```python
from build123d import *

# Parameters (mm, degrees)
SKETCH2_R           = 39.5
BOSS_EXTRUDE1_DEPTH = 1
SKETCH4_R           = 41.25
BOSS_EXTRUDE2_DEPTH = 1
SKETCH5_R           = 42
BOSS_EXTRUDE3_DEPTH = 7
SKETCH6_R           = 35
BOSS_EXTRUDE4_DEPTH = 7
BOSS_EXTRUDE5_DEPTH = 3
CIRPATTERN1_COUNT   = 12
SKETCH8_R           = 15
BOSS_EXTRUDE6_DEPTH = 10
SKETCH9_W           = 35
SKETCH9_H           = 40
BOSS_EXTRUDE7_DEPTH = 42
BOSS_EXTRUDE8_DEPTH = 35
SKETCH11_R          = 15
BOSS_EXTRUDE9_DEPTH = 10


with BuildPart() as part:
    # Sketch1 → Revolve1 (revolve)
    with BuildSketch(Plane.XY):
        with BuildLine():
            Line((-35, 0), (0, 0))
            Line((0, 0), (0, -20))
            Line((0, -20), (-40, -20))
            ThreePointArc((-40, -20), (-39.657515479, -9.46062113), (-35, 0))
        make_face()
    revolve(axis=Axis((0, 0, 0), (0, -1, 0)))

    # Sketch2 → Boss-Extrude1 (add)
    with BuildSketch(Plane.XZ.offset(20)):
        Circle(SKETCH2_R)
    extrude(amount=BOSS_EXTRUDE1_DEPTH)

    # Sketch3 → Revolve2 (revolve)
    with BuildSketch(Plane(origin=(0, 0, 0), x_dir=(0, 0, -1), z_dir=(1, 0, 0))):
        with BuildLine():
            Line((0, -21), (-40, -21))
            ThreePointArc((-40, -21), (-42.384109041, -30.861589096), (-42, -41))
            Line((-42, -41), (0, -41))
            Line((0, -41), (0, -21))
        make_face()
    revolve(axis=Axis((0, -21, 0), (0, -1, 0)))

    # Sketch4 → Boss-Extrude2 (add)
    with BuildSketch(Plane.XZ.offset(41)):
        Circle(SKETCH4_R)
    extrude(amount=BOSS_EXTRUDE2_DEPTH)

    # Sketch5 → Boss-Extrude3 (add)
    with BuildSketch(Plane.XZ.offset(42)):
        Circle(SKETCH5_R)
    extrude(amount=BOSS_EXTRUDE3_DEPTH)

    # Sketch6 → Boss-Extrude4 (add)
    with BuildSketch(Plane.XZ.offset(49)):
        Circle(SKETCH6_R)
    extrude(amount=BOSS_EXTRUDE4_DEPTH)

    # Sketch7 → Boss-Extrude5 (add)
    with BuildSketch(Plane.XZ.offset(49)):
        Polygon((40.75, 0), (39.625, 1.948557159), (37.375, 1.948557159), (36.25, 0), (37.375, -1.948557159), (39.625, -1.948557159), align=None)
        Polygon((39.047649731, 0.948557159), (37.952350269, 0.948557159), (37.404700538, 0), (37.952350269, -0.948557159), (39.047649731, -0.948557159), (39.595299462, 0), align=None, mode=Mode.SUBTRACT)
    boss_extrude5 = extrude(amount=BOSS_EXTRUDE5_DEPTH)

    # CirPattern1: Boss-Extrude5 ×12 about axis
    cirpattern1_axis = Axis((0, 0, 0), (0, 1, 0))
    for i in range(1, CIRPATTERN1_COUNT):
        add(boss_extrude5.rotate(cirpattern1_axis, i * 360 / CIRPATTERN1_COUNT))

    # Sketch8 → Boss-Extrude6 (add)
    with BuildSketch(Plane.XZ.offset(56)):
        Circle(SKETCH8_R)
    extrude(amount=BOSS_EXTRUDE6_DEPTH)

    # Sketch9 → Boss-Extrude7 (add)
    with BuildSketch(Plane(origin=(0, 0, 0), x_dir=(1, 0, 0), z_dir=(0, 1, 0))):
        Rectangle(SKETCH9_W, SKETCH9_H)
    extrude(amount=BOSS_EXTRUDE7_DEPTH)

    # Sketch10 → Boss-Extrude8 (add)
    with BuildSketch(Plane.ZY.offset(17.5)):
        with BuildLine():
            Line((-20, 42), (20, 42))
            ThreePointArc((20, 42), (0, 62), (-20, 42))
        make_face()
    extrude(amount=-BOSS_EXTRUDE8_DEPTH)

    # Sketch11 → Boss-Extrude9 (add)
    with BuildSketch(Plane.ZY.offset(17.5)):
        with Locations((0, 42)):
            Circle(SKETCH11_R)
    boss_extrude9 = extrude(amount=BOSS_EXTRUDE9_DEPTH)

    # Mirror1: Boss-Extrude9 across plane
    add(boss_extrude9.mirror(Plane(origin=(0, 0, 0), x_dir=(0, 0, 1), z_dir=(1, 0, 0))))


solid = part.part
```
Check sheet for the modelled part. Datum: model origin and axes. Units: mm. A direction names the side the tool comes from. Give positions to 0.01 mm unless a question says otherwise; leave off trailing zeros. Loops run counter-clockwise (first coordinate to the right, second up) from the corner with the lowest first, then second, coordinate; pieces in that order, holes last. Notation, with made-up numbers: M 18.5,84.5 L 39.5,84.5 A23 ccw 39.5,99.5 Z; hole C 65.25,56 d6. An arc over 180 degrees is marked long. Answer as CSV lines item,"result".
Item 1: Depth check by flat-ended pin: pin 1 Ø10 at (x, z) = (13, -17.5) entering from +Y; pin 2 Ø1.2 at (x, z) = (-32.5, 19.5) entering from -Y; pin 3 Ø3 at (x, z) = (-7.5, 5.5) entering from +Y. Enter the tip coordinate at first touch or a pass-through.
Reply:
pin 1,"y = 57.61"
pin 2,"y = -52"
pin 3,"y = 61.6"
Item 2: Draft check along X on faces 5 (the face through (-29.11, -20.49, 26.7)), 6 (the face through (20.5, -52, -33.7)). Enter one of: pulls with the +X half, pulls with the -X half, needs draft (parallel to the pull), parting line crosses it, or undercut.
Reply:
face 5,"parting line crosses it"
face 6,"needs draft"
Item 3: Sectioned sample at A-A, the plane y = -46. Enter the section's corners in (x, z), then the cut area to 3 significant figures.
Reply:
outline,"C 0,0 d84"
area,"5,540 mm^2"
Item 4: Scan lines: L1, parallel to Z at x = 8, y = 30; L2, parallel to Y at x = 10, z = -31.5; L3, parallel to X at y = 45, z = 12.5. Record each from-to range of solid material in increasing order.
Reply:
L1,"-20 to 20"
L2,"-56 to 0"
L3,"-27.5 to 27.5"
Item 5: Set-up check for faces 1 (the face through (-22.43, 56.872, -1.953)), 2 (the face through (33.7, -52, 20.5)), 3 (the face through (28, -42, -31)), 4 (the face through (15, -56, -7)): record each of +Z, -Z, +X, -X, +Y, -Y from which the full face is reachable in a straight line by a thin tool's end or side.
Reply:
face 1,"-X"
face 2,"+Z, +X, -Y"
face 3,"none"
face 4,"-Y"
